Design review of the part shown in the three views and the two pictorial views. Dimensions are in mm from the part's minimum x, y and z. Coordinates: 2 decimals unless noted, no trailing zeros. Loops run counter-clockwise (first coordinate to the right, second up) from the corner with the lowest first, then second, coordinate; pieces in that order, holes last. Notation, with made-up numbers: M -33,50.5 L -21,50.5 A12 cw -21,63.5 Z; hole C 12.5,66.5 d7. An arc over 180 degrees is marked long. Use one line per item in the form item = value.
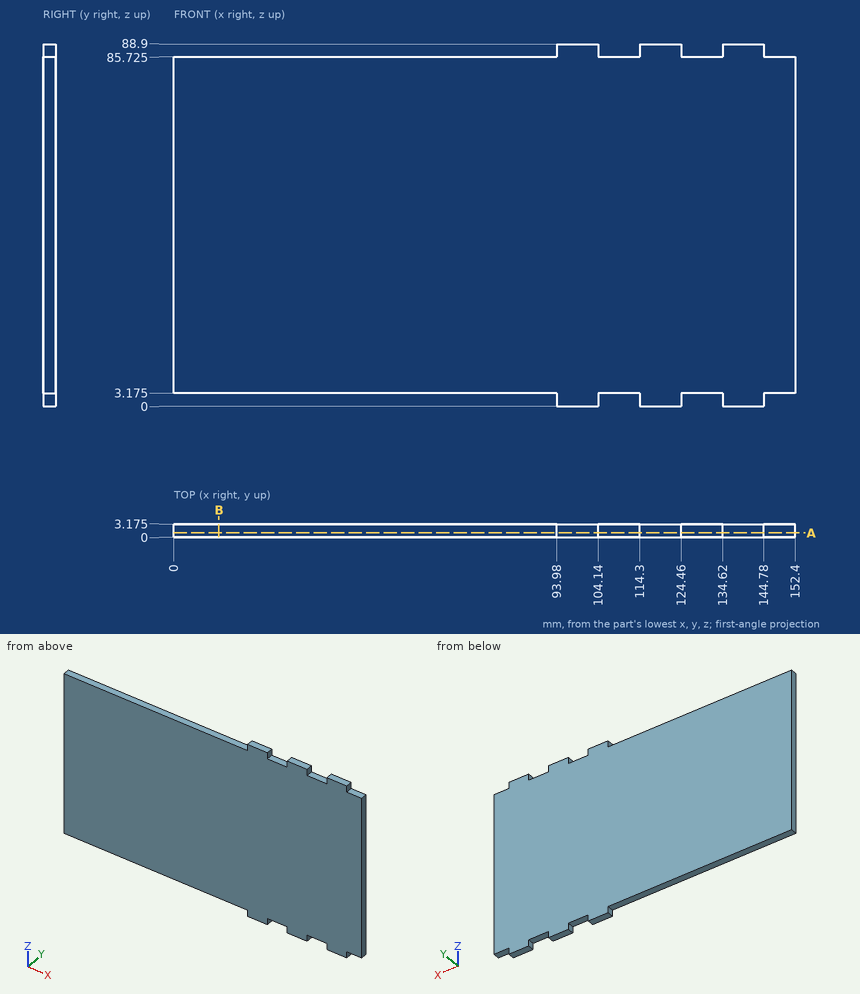
1. Add section A-A (y = 1.05). State the section outline as (x, z) points (3 decimals), then the cut area to 3 significant figures.
Response values:
outline = M 0,3.175 L 93.98,3.175 L 93.98,0 L 104.14,0 L 104.14,3.175 L 114.3,3.175 L 114.3,0 L 124.46,0 L 124.46,3.175 L 134.62,3.175 L 134.62,0 L 144.78,0 L 144.78,3.175 L 152.4,3.175 L 152.4,85.725 L 144.78,85.725 L 144.78,88.9 L 134.62,88.9 L 134.62,85.725 L 124.46,85.725 L 124.46,88.9 L 114.3,88.9 L 114.3,85.725 L 104.14,85.725 L 104.14,88.9 L 93.98,88.9 L 93.98,85.725 L 0,85.725 Z
area = 12,800 mm^2
2. Wall thickness on line 1 along Z through (x, y) = (29, 0.3) (3 decimals): over which ranges is the line inside the solid? List them lowest first. Write a range as from..to.
Response values:
line_1 = 3.175..85.725
3. Add section B-B (x = 11). State the section outline as (y, z) points (3 decimals).
Response values:
outline = M 0,3.175 L 3.175,3.175 L 3.175,85.725 L 0,85.725 Z
4. Insertion check: P1, Ø1, axis at x = 123.5, z = 23.5, coming from the -Y side; P2, Ø1.6, axis at y = 2.5, z = 87.5, coming from the -X side; P3, Ø1, axis at x = 149.5, y = 1.5, coming from the +Z side (3 decimals). Each pin has a flat end and moves straight along its axis. Give the tip position at first contact, or say it passes through.
Response values:
P1 = 0
P2 = 93.98
P3 = 85.725
